```python
from build123d import *

# Parameters (mm, degrees)
SKETCH1_R           = 76.2
SKETCH1_R_2         = 4.5
SKETCH1_R_3         = 55
BOSS_EXTRUDE1_DEPTH = 3
SKETCH2_R           = 3.1
CUT_EXTRUDE1_DEPTH  = 3


with BuildPart() as part:
    # Sketch1 → Boss-Extrude1 (new body)
    with BuildSketch(Plane(origin=(0, 0, 0), x_dir=(1, 0, 0), z_dir=(0, 1, 0))):
        with Locations(Location((0, 0, 0), (0, 0, 270))):
            Circle(SKETCH1_R)
        with Locations(Location((0, 62.5, 0), (0, 0, 270))):
            Circle(SKETCH1_R_2, mode=Mode.SUBTRACT)
        with Locations(Location((62.5, 0, 0), (0, 0, 270))):
            Circle(SKETCH1_R_2, mode=Mode.SUBTRACT)
        with Locations(Location((0, -62.5, 0), (0, 0, 270))):
            Circle(SKETCH1_R_2, mode=Mode.SUBTRACT)
        with Locations(Location((-62.5, 0, 0), (0, 0, 270))):
            Circle(SKETCH1_R_2, mode=Mode.SUBTRACT)
        with Locations(Location((0, 0, 0), (0, 0, 270))):
            Circle(SKETCH1_R_3, mode=Mode.SUBTRACT)
    extrude(amount=BOSS_EXTRUDE1_DEPTH)

    # Sketch2 → Cut-Extrude1 (cut)
    with BuildSketch(Plane(origin=(0, 3, 0), x_dir=(1, 0, 0), z_dir=(0, 1, 0))):
        with Locations(Location((-51.618795027, 37.476659403, 0), (0, 0, 270))):
            Circle(SKETCH2_R)
        with Locations(Location((-37.476659403, 51.618795027, 0), (0, 0, 270))):
            Circle(SKETCH2_R)
    extrude(amount=-CUT_EXTRUDE1_DEPTH, mode=Mode.SUBTRACT)


solid = part.part
```
Work out the finished part from the listing and answer in its coordinate system (mm). Give positions to 0.01 mm unless a question says otherwise; leave off trailing zeros. Order: outer loops, then holes, each group sorted by start corner. A loop starts at its lowest first (then second) coordinate and runs counter-clockwise, first axis right, second up. Notation, with made-up numbers: M 23,-13 L 29,-13 A33 cw 29,16 Z; hole C 22,-14 d5. An arc over 180 degrees is marked long. Return JSON: item names as keys, results as strings.
1) Section D-D, the plane x = 25.5 is taken. Write down the section's boundary in (y, z), plus the area to 3 significant figures.
Resolved:
{"outline": "M 0,-71.81 L 3,-71.81 L 3,-48.73 L 0,-48.73 Z; M 0,48.73 L 3,48.73 L 3,71.81 L 0,71.81 Z", "area": "138 mm^2"}
2) Section A-A, the plane z = 0 is taken. Write down the section's boundary in (x, y).
Resolved:
{"outline": "M -76.2,0 L -67,0 L -67,3 L -76.2,3 Z; M -58,0 L -55,0 L -55,3 L -58,3 Z; M 55,0 L 58,0 L 58,3 L 55,3 Z; M 67,0 L 76.2,0 L 76.2,3 L 67,3 Z"}
3) For a pull along X with two mould halves and no side action, classify faces 1 (the flat face through (22.9, 0, 50.4)), 2 (the cylindrical face through (-46.367, 1.479, -60.47)), 3 (the cylindrical face through (-48.794, 1.479, 25.379)) as +X half, -X half, draft (parallel to the pull), parting line (faces both ways), or undercut.
Resolved:
{"face 1": "draft", "face 2": "parting line", "face 3": "undercut"}
4) Section C-C, the plane z = 31.5 is taken. Write down the section's boundary in (x, y), plus the area to 3 significant figures.
Resolved:
{"outline": "M -69.38,0 L -45.09,0 L -45.09,3 L -69.38,3 Z; M 45.09,0 L 69.38,0 L 69.38,3 L 45.09,3 Z", "area": "146 mm^2"}
5) Section B-B, the plane x = 0 is taken. Write down the section's boundary in (y, z).
Resolved:
{"outline": "M 0,-76.2 L 3,-76.2 L 3,-67 L 0,-67 Z; M 0,-58 L 3,-58 L 3,-55 L 0,-55 Z; M 0,55 L 3,55 L 3,58 L 0,58 Z; M 0,67 L 3,67 L 3,76.2 L 0,76.2 Z"}
6) Straight lines are drawn through the part: line 1 along X through (y, z) = (0.95, 0); line 2 along Z through (x, y) = (2, 1.15); line 3 along X through (y, z) = (0.7, -35). For each, find the intervals that lie inside material, in ascending order. Write a range as [from, to].
Resolved:
{"line 1": "[-76.2, -67], [-58, -55], [55, 58], [67, 76.2]", "line 2": "[-76.17, -66.53], [-58.47, -54.96], [54.96, 58.47], [66.53, 76.17]", "line 3": "[-67.69, -53.48], [-49.75, -42.43], [42.43, 67.69]"}
